Geometry check sheet. Reference: the model listing, model coordinates, mm. Face numbers are marked on the shaded views. Round coordinates to 2 decimals unless told otherwise and drop trailing zeros. Loops run counter-clockwise (first coordinate to the right, second up) from the corner with the lowest first, then second, coordinate; pieces in that order, holes last. Notation, with made-up numbers: M 56,56 L 101,56 A5 cw 101,65 Z; hole C 43.5,-14 d7. An arc over 180 degrees is marked long. Write item = value, one per line.
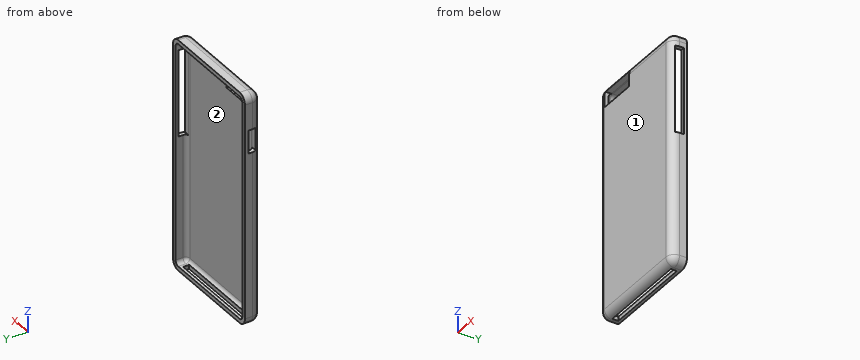
from build123d import *

# Parameters (mm, degrees)
F0_W        = 69.596
F0_H        = 140.716
F1_DEPTH    = 9.652
F2_R        = 5.08
F3_T1_DEPTH = 17.272
F3_S5_W     = 5.08
F3_S5_H     = 5.08
F3_T6_DEPTH = 5.08
F4_T1_DEPTH = 17.272
F4_S5_W     = 5.08
F4_S5_H     = 5.08
F4_T6_DEPTH = 5.08
F5_T1_DEPTH = 17.272
F5_S5_W     = 5.08
F5_S5_H     = 5.08
F5_T6_DEPTH = 5.08
F6_T        = -2.54
F7_W        = 23.9500291884
F7_H        = 9.7231566906
F8_DEPTH    = 25.4
F9_W        = 5.1087748725
F9_H        = 52.7357356623
F10_DEPTH   = 25.4
F11_W       = 4.6143759973
F11_H       = 14.0079259872
F12_DEPTH   = 25.4
F14_W       = 56.6909182817
F14_H       = 3.6255817395
F15_DEPTH   = 25.4


# Not quite as in the source:
# - a fillet or chamfer that OpenCascade refuses, or shapes differently, is made with other operations: its cross-section is extruded or revolved along the edge and cut away or added


with BuildPart() as f1:
    # F0 (on Front) → F1 (new body)
    with BuildSketch(Plane.XZ):
        Rectangle(F0_W, F0_H)
    extrude(amount=F1_DEPTH)

    # F2
    f2_edges = [f1.edges().sort_by_distance(p)[0] for p in [
        (-34.798, -4.826, 70.358),
        (0, -9.652, 70.358),
        (-34.798, -9.652, 0),
        (0, -9.652, -70.358),
        (34.798, -9.652, 0),
    ]]
    fillet(f2_edges, radius=F2_R)

    # F3: fillet of radius 5.08 on 1 edges, made by hand

    # F3_s2 → F3_t1 (cut)
    with BuildSketch(Plane.XZ.offset(-12.7)):
        with BuildLine():
            ThreePointArc((29.718, 70.358), (33.3101024484, 68.8701024484), (34.798, 65.278))
            Line((34.798, 65.278), (34.798, 70.358))
            Line((34.798, 70.358), (29.718, 70.358))
        make_face()
    extrude(amount=F3_T1_DEPTH, mode=Mode.SUBTRACT)


with BuildPart() as f3_tool4:
    # F3_s5 → F3_t6 (new body)
    with BuildSketch(Plane.XY.offset(65.278)):
        with Locations((32.258, -7.112)):
            Rectangle(F3_S5_W, F3_S5_H)
    extrude(amount=F3_T6_DEPTH)

    # F3_s7 → F3_t8 (revolve, cut)
    with BuildSketch(Plane(origin=(29.718, -4.572, 65.278), x_dir=(-0.7071067812, 0.7071067812, 0), z_dir=(0.7071067812, 0.7071067812, 0))):
        with BuildLine():
            ThreePointArc((0, -5.08), (5.08, 0), (0, 5.08))
            Line((0, 5.08), (0, -5.08))
        make_face()
    revolve(axis=Axis((29.718, -4.572, 65.278), (0, 0, 1)), mode=Mode.SUBTRACT)


with BuildPart() as f1_1:
    add(f1.part)

    # F3_t3: cut F3_tool4
    add(f3_tool4.part, mode=Mode.SUBTRACT)

    # F4: fillet of radius 5.08 on 1 edges, made by hand

    # F4_s2 → F4_t1 (cut)
    with BuildSketch(Plane.XZ.offset(-12.7)):
        with BuildLine():
            ThreePointArc((-29.718, -70.358), (-33.3101024484, -68.8701024484), (-34.798, -65.278))
            Line((-34.798, -65.278), (-34.798, -70.358))
            Line((-34.798, -70.358), (-29.718, -70.358))
        make_face()
    extrude(amount=F4_T1_DEPTH, mode=Mode.SUBTRACT)


with BuildPart() as f4_tool4:
    # F4_s5 → F4_t6 (new body)
    with BuildSketch(Plane.XY.offset(-65.278)):
        with Locations((-32.258, -7.112)):
            Rectangle(F4_S5_W, F4_S5_H)
    extrude(amount=-F4_T6_DEPTH)

    # F4_s7 → F4_t8 (revolve, cut)
    with BuildSketch(Plane(origin=(-29.718, -4.572, -65.278), x_dir=(0.7071067812, 0.7071067812, 0), z_dir=(-0.7071067812, 0.7071067812, 0))):
        with BuildLine():
            ThreePointArc((0, -5.08), (5.08, 0), (0, 5.08))
            Line((0, 5.08), (0, -5.08))
        make_face()
    revolve(axis=Axis((-29.718, -4.572, -65.278), (0, 0, -1)), mode=Mode.SUBTRACT)


with BuildPart() as f1_2:
    add(f1_1.part)

    # F4_t3: cut F4_tool4
    add(f4_tool4.part, mode=Mode.SUBTRACT)

    # F5: fillet of radius 5.08 on 1 edges, made by hand

    # F5_s2 → F5_t1 (cut)
    with BuildSketch(Plane.XZ.offset(-12.7)):
        with BuildLine():
            ThreePointArc((34.798, -65.278), (33.3101024484, -68.8701024484), (29.718, -70.358))
            Line((29.718, -70.358), (34.798, -70.358))
            Line((34.798, -70.358), (34.798, -65.278))
        make_face()
    extrude(amount=F5_T1_DEPTH, mode=Mode.SUBTRACT)


with BuildPart() as f5_tool4:
    # F5_s5 → F5_t6 (new body)
    with BuildSketch(Plane.YZ.offset(29.718)):
        with Locations((-7.112, -67.818)):
            Rectangle(F5_S5_W, F5_S5_H)
    extrude(amount=F5_T6_DEPTH)

    # F5_s7 → F5_t8 (revolve, cut)
    with BuildSketch(Plane(origin=(29.718, -4.572, -65.278), x_dir=(0, 0.7071067812, 0.7071067812), z_dir=(0, 0.7071067812, -0.7071067812))):
        with BuildLine():
            ThreePointArc((0, -5.08), (5.08, 0), (0, 5.08))
            Line((0, 5.08), (0, -5.08))
        make_face()
    revolve(axis=Axis((29.718, -4.572, -65.278), (1, 0, 0)), mode=Mode.SUBTRACT)


with BuildPart() as f1_3:
    add(f1_2.part)

    # F5_t3: cut F5_tool4
    add(f5_tool4.part, mode=Mode.SUBTRACT)

    # F6
    f6_openings = [f1_3.faces().sort_by_distance(p)[0] for p in [
        (0, 0, 0),
    ]]
    offset(amount=F6_T, openings=f6_openings)

    # F7 (on face) → F8 (cut)
    with BuildSketch(Plane.XZ.offset(9.652)):
        with Locations((-17.7429854058, 62.7884864807)):
            Rectangle(F7_W, F7_H)
    extrude(amount=-F8_DEPTH, mode=Mode.SUBTRACT)

    # F9 (on face) → F10 (cut)
    with BuildSketch(Plane.YZ.offset(34.798)):
        with Locations((-4.3671781896, 35.8438207768)):
            Rectangle(F9_W, F9_H)
    extrude(amount=-F10_DEPTH, mode=Mode.SUBTRACT)

    # F11 (on face) → F12 (cut)
    with BuildSketch(Plane(origin=(-34.798, 0, 0), x_dir=(0, -1, 0), z_dir=(-1, 0, 0))):
        with Locations((4.6143762302, 42.0237891376)):
            Rectangle(F11_W, F11_H)
    extrude(amount=-F12_DEPTH, mode=Mode.SUBTRACT)

    # F14 (on face) → F15 (cut)
    with BuildSketch(Plane(origin=(0, 0, -70.358), x_dir=(1, 0, 0), z_dir=(0, 0, -1))):
        with Locations((-0.3109676763, 3.6884165602)):
            Rectangle(F14_W, F14_H)
    extrude(amount=-F15_DEPTH, mode=Mode.SUBTRACT)


solid = f1_3.part
(1) Sectioned sample at B-B on z = 18.5. Record the cut outline in (x, y), then the cut area to 3 significant figures.
Result set:
outline = M -34.8,-4.57 A5.08 ccw -29.72,-9.65 L 29.72,-9.65 A5.08 ccw 34.22,-6.92 L 30.68,-6.92 A2.54 cw 29.72,-7.11 L -29.72,-7.11 A2.54 cw -32.26,-4.57 L -32.26,0 L -34.8,0 Z; M 32.26,-1.81 L 34.8,-1.81 L 34.8,0 L 32.26,0 Z
area = 191 mm2
(2) Material ranges on line 1 along X through (y, z) = (-3, 5); line 2 along Z through (x, y) = (11, -3.25); line 3 along Y through (x, z) = (24, 2.5), recorded low to high. Write a range as from..to.
Result set:
line_1 = -34.8..-32.26, 32.26..34.8
line_2 = 67.82..70.36
line_3 = -9.65..-7.11
(3) Release check for a two-part mould opening along X. For the marked faces 1 and 2 record: released by +X, released by -X, zero draft, split by the parting line, or undercut.
Result set:
face_1 = zero draft
face_2 = undercut
(4) Sectioned sample at C-C on x = 15.5. Record the cut outline in (y, z).
Result set:
outline = M -9.65,-65.28 A5.08 ccw -5.5,-70.27 L -5.5,-67.64 A2.54 cw -7.11,-65.28 L -7.11,65.28 A2.54 cw -4.57,67.82 L 0,67.82 L 0,70.36 L -4.57,70.36 A5.08 ccw -9.65,65.28 Z; M -1.88,-70.36 L 0,-70.36 L 0,-67.82 L -1.88,-67.82 Z
(5) Depth check by flat-ended pin: pin 1 Ø1.5 at (x, y) = (-4.5, -4) entering from -Z; pin 2 Ø5 at (y, z) = (-7.5, 43.5) entering from +X; pin 3 Ø1.2 at (x, y) = (-33, -5) entering from -Z. Enter the tip coordinate at first touch or a pass-through.
Result set:
pin_1 = 67.81
pin_2 = 34.22
pin_3 = -69.57
(6) Sectioned sample at A-A on x = -18.5. Record the cut outline in (y, z), then the cut area to 3 significant figures.
Result set:
outline = M -9.65,-65.28 A5.08 ccw -5.5,-70.27 L -5.5,-67.64 A2.54 cw -7.11,-65.28 L -7.11,57.93 L -9.65,57.93 Z; M -9.06,67.65 L -5.48,67.65 A2.54 cw -4.57,67.82 L 0,67.82 L 0,70.36 L -4.57,70.36 A5.08 ccw Z; M -1.88,-70.36 L 0,-70.36 L 0,-67.82 L -1.88,-67.82 Z
area = 351 mm2
(7) Sectioned sample at D-D on z = -18.5. Record the cut outline in (x, y).
Result set:
outline = M -34.8,-4.57 A5.08 ccw -29.72,-9.65 L 29.72,-9.65 A5.08 ccw 34.8,-4.57 L 34.8,0 L 32.26,0 L 32.26,-4.57 A2.54 cw 29.72,-7.11 L -29.72,-7.11 A2.54 cw -32.26,-4.57 L -32.26,0 L -34.8,0 Z
